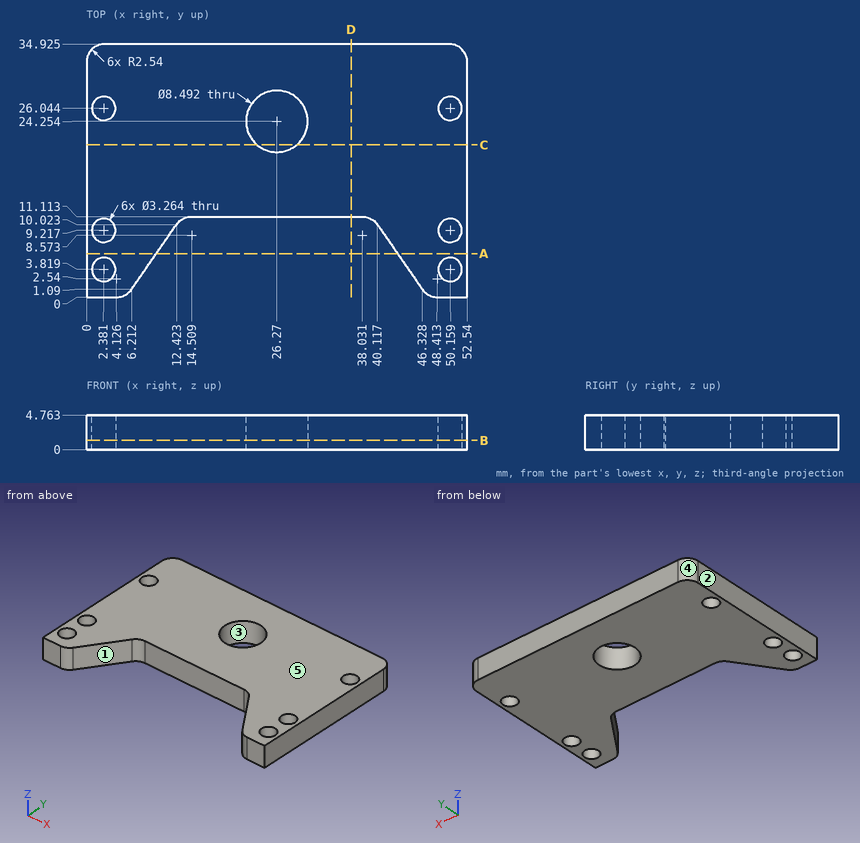
The drawing under review shows one solid part. Ordinate dimensions are in mm from its lowest x, y, z. A direction names the side the tool comes from. Give positions to 0.01 mm unless a question says otherwise; leave off trailing zeros. Order: outer loops, then holes, each group sorted by start corner. A loop starts at its lowest first (then second) coordinate and runs counter-clockwise, first axis right, second up. Notation, with made-up numbers: M -11,26.5 L 5,26.5 A8 cw 5,38.5 Z; hole C 46.25,16.25 d6. An arc over 180 degrees is marked long. Answer in a Markdown table with one row per item. Add a question column.
1. Add section D-D on x = 36.5. State the section outline as (y, z) points (1 decimal).
2. To check wall thickness, follow line 1 along Y through (x, z) = (50, 3.8) (1 decimal); line 2 along Y through (x, z) = (49, 2.55) (1 decimal); line 3 along Y through (x, z) = (26, 0.55) (1 decimal). State the ranges of each line that lie inside material, in increasing order.
3. Mouldability with a two-part tool opening along X and no side actions: class the marked faces 3, 4 and 5 as released by +X, released by -X, zero draft, split by the parting line, or undercut.
4. For pin 1 Ø5 at (x, y) = (26.27, 24.25) entering from -Z, flat-tipped, find the tip position at first contact; note if it passes through.
5. Add section B-B on z = 1.3. Count the separate pieces of the cut face and the enclosed holes in it, plus the area to 3 significant figures.
6. Add section A-A on y = 6. State the section outline as (x, z) points.
7. Add section C-C on y = 21. State the section outline as (x, z) points, plus the area to 3 significant figures.
8. Machinability: for the marked faces 1 and 2, which of the approach directions +Z, -Z, +X, -X, +Y, -Y give a long, thin tool a straight path to every point of the face, cutting with its end or side? Answer none if there is none.
The answers:
| question | item | result |
|---|---|---|
| 1 | outline | M 11.1,0 L 34.9,0 L 34.9,4.8 L 11.1,4.8 Z |
| 2 | line 1 | 0 to 2.2, 5.4 to 7.6, 10.8 to 24.4, 27.7 to 34.9 |
| 2 | line 2 | 0 to 2.7, 5 to 8.1, 10.4 to 24.9, 27.2 to 34.9 |
| 2 | line 3 | 11.1 to 20, 28.5 to 34.9 |
| 3 | face 3 | undercut |
| 3 | face 4 | released by -X |
| 3 | face 5 | zero draft |
| 4 | pin 1 | through |
| 5 | separate pieces | 1 |
| 5 | enclosed holes | 7 |
| 5 | area | 1,350 mm2 |
| 6 | outline | M 0,0 L 9.63,0 L 9.63,4.76 L 0,4.76 Z; M 42.91,0 L 52.54,0 L 52.54,4.76 L 42.91,4.76 Z |
| 7 | outline | M 0,0 L 23.54,0 L 23.54,4.76 L 0,4.76 Z; M 29,0 L 52.54,0 L 52.54,4.76 L 29,4.76 Z |
| 7 | area | 224 mm2 |
| 8 | face 1 | +Z, -Z, -Y |
| 8 | face 2 | +Z, -Z, -X, +Y, -Y |
